```python
from build123d import *

# Parameters (mm, degrees)
SKETCH1_R                 = 11
BOSS_EXTRUDE1_DEPTH       = 2
SKETCH3_R                 = 3.5
BOSS_EXTRUDE2_DEPTH       = 2
M2X0_4_TAPPED_HOLE1_D     = 1.6
M2X0_4_TAPPED_HOLE1_DEPTH = 5.2
M2X0_4_TAPPED_HOLE1_TIP   = 0.480688495
SKETCH8_R                 = 2
SKETCH8_R_2               = 1.25
BOSS_EXTRUDE3_DEPTH       = 1
M3X0_5_TAPPED_HOLE1_D     = 2.5
M3X0_5_TAPPED_HOLE1_DEPTH = 7.5
M3X0_5_TAPPED_HOLE1_TIP   = 0.751075774


with BuildPart() as part:
    # Sketch1 → Boss-Extrude1 (new body)
    with BuildSketch(Plane.XY):
        Circle(SKETCH1_R)
    extrude(amount=BOSS_EXTRUDE1_DEPTH)

    # Sketch3 → Boss-Extrude2 (add)
    with BuildSketch(Plane.XY.offset(2)):
        Circle(SKETCH3_R)
    extrude(amount=BOSS_EXTRUDE2_DEPTH)

    # M2x0.4 Tapped Hole1
    with Locations(Plane.XY.offset(2)):
        with Locations((0, 8), (-5.656854249, 5.656854249), (-8, 0), (-5.656854249, -5.656854249), (0, -8), (5.656854249, -5.656854249), (8, 0), (5.656854249, 5.656854249)):
            Hole(M2X0_4_TAPPED_HOLE1_D / 2, depth=M2X0_4_TAPPED_HOLE1_DEPTH)
            with Locations((0, 0, -(M2X0_4_TAPPED_HOLE1_DEPTH + M2X0_4_TAPPED_HOLE1_TIP / 2))):  # 118° drill point
                Cone(0, M2X0_4_TAPPED_HOLE1_D / 2, M2X0_4_TAPPED_HOLE1_TIP, mode=Mode.SUBTRACT)

    # Sketch8 → Boss-Extrude3 (add)
    with BuildSketch(Plane(origin=(0, 0, 0), x_dir=(-1, 0, 0), z_dir=(0, 0, -1))):
        Circle(SKETCH8_R)
        Circle(SKETCH8_R_2, mode=Mode.SUBTRACT)
    extrude(amount=BOSS_EXTRUDE3_DEPTH)

    # M3x0.5 Tapped Hole1
    with Locations(Plane.XY.offset(4)):
        with Locations((0, 0)):
            Hole(M3X0_5_TAPPED_HOLE1_D / 2, depth=M3X0_5_TAPPED_HOLE1_DEPTH)
            with Locations((0, 0, -(M3X0_5_TAPPED_HOLE1_DEPTH + M3X0_5_TAPPED_HOLE1_TIP / 2))):  # 118° drill point
                Cone(0, M3X0_5_TAPPED_HOLE1_D / 2, M3X0_5_TAPPED_HOLE1_TIP, mode=Mode.SUBTRACT)


solid = part.part
```
Model file for the job. Use its own axes, mm. A direction names the side the tool comes from. Coordinates: 2 decimals unless noted, no trailing zeros. Order: outer loops, then holes, each group sorted by start corner. A loop starts at its lowest first (then second) coordinate and runs counter-clockwise, first axis right, second up. Notation, with made-up numbers: (70.5, -5.5) -> (127.5, -5.5) arc R27 cw to (127.5, 17.5) -> close; hole circle Ø4 at (56, 38). An arc over 180 degrees is marked (long way). Return JSON: item names as keys, results as strings.
Item 1: Wall check: line 1 along Y through (x, z) = (0, 1.25); line 2 along Y through (x, z) = (0, 2.8); line 3 along Y through (x, z) = (0, -0.45). Give the ranges that are in metal, low to high. Write a range as from..to.
Model answer:
{"line 1": "y = -11..-8.8, -7.2..-1.25, 1.25..7.2, 8.8..11", "line 2": "y = -3.5..-1.25, 1.25..3.5", "line 3": "y = -2..-1.25, 1.25..2"}
Item 2: Mould opens along Y. For faces 1 (the face through (0.434, -1.952, -0.493)), 2 (the face through (-3, 3, 2)), 3 (the face through (6.456, -5.622, 0.986)) say: pulls with the +Y half, pulls with the -Y half, needs draft (parallel to the pull), parting line crosses it, or undercut.
Model answer:
{"face 1": "parting line crosses it", "face 2": "needs draft", "face 3": "undercut"}
Item 3: 3-axis set-ups, long thin cutter, end or side, ignore diameter. For faces 4 (the face through (-6.396, 5.35, 0.986)), 5 (the face through (3.233, -1.341, 2.986)): which of +Z, -Z, +X, -X, +Y, -Y reach the whole face in a straight line?
Model answer:
{"face 4": "+Z, -Z", "face 5": "+Z"}
Item 4: Slice it at A-A (y = 0). Write the cut outline in (x, z), then the cut area to 3 significant figures.
Model answer:
{"outline": "(-11, 0) -> (-8.8, 0) -> (-8.8, 2) -> (-11, 2) -> close; (-7.2, 0) -> (-2, 0) -> (-2, -1) -> (-1.25, -1) -> (-1.25, 4) -> (-3.5, 4) -> (-3.5, 2) -> (-7.2, 2) -> close; (1.25, -1) -> (2, -1) -> (2, 0) -> (7.2, 0) -> (7.2, 2) -> (3.5, 2) -> (3.5, 4) -> (1.25, 4) -> close; (8.8, 0) -> (11, 0) -> (11, 2) -> (8.8, 2) -> close", "area": "43.1 mm²"}
Item 5: Pin check, flat tips, straight feed: P1, Ø1.8, axis at x = 0, y = 8, coming from the -Z side; P2, Ø1.5, axis at x = 0, y = 0, coming from the +Z side; P3, Ø3, axis at x = 0, y = 0, coming from the -Z side; P4, Ø2, axis at x = -8, y = 0, coming from the +Z side. Stop position of each tip, or through.
Model answer:
{"P1": "stops at z = 0", "P2": "passes through", "P3": "stops at z = -1", "P4": "stops at z = 2"}
Item 6: Slice it at B-B (x = -8.5). Write the cut outline in (y, z).
Model answer:
{"outline": "(-6.98, 0) -> (-0.62, 0) -> (-0.62, 2) -> (-6.98, 2) -> close; (0.62, 0) -> (6.98, 0) -> (6.98, 2) -> (0.62, 2) -> close"}
Item 7: Slice it at D-D (z = 1.45). Count the separate pieces of the cut face and the enclosed holes in it, then the cut area to 3 significant figures.
Model answer:
{"separate pieces": "1", "enclosed holes": "9", "area": "359 mm²"}
